from build123d import *

# Parameters (mm, degrees)
SKETCH1_W           = 13
SKETCH1_H           = 30
SKETCH1_R           = 1.8
BOSS_EXTRUDE1_DEPTH = 3
SKETCH2_W           = 13
SKETCH2_H           = 7
BOSS_EXTRUDE2_DEPTH = 31.69
SKETCH3_W           = 10
SKETCH3_H           = 14
CUT_EXTRUDE1_DEPTH  = 5.5
SKETCH4_W           = 3
SKETCH4_H           = 4
CUT_EXTRUDE2_DEPTH  = 47.940346185
FILLET1_R           = 3


with BuildPart() as part:
    # Sketch1 → Boss-Extrude1 (new body)
    with BuildSketch(Plane.XY):
        with Locations((6.5, 15)):
            Rectangle(SKETCH1_W, SKETCH1_H)
        with Locations((6.5, 25.2)):
            Circle(SKETCH1_R, mode=Mode.SUBTRACT)
        with Locations((6.5, 4.8)):
            Circle(SKETCH1_R, mode=Mode.SUBTRACT)
    extrude(amount=BOSS_EXTRUDE1_DEPTH)

    # Sketch2 → Boss-Extrude2 (add)
    with BuildSketch(Plane.XY.offset(3)):
        with Locations((6.5, 15)):
            Rectangle(SKETCH2_W, SKETCH2_H)
    extrude(amount=BOSS_EXTRUDE2_DEPTH)

    # Sketch3 → Cut-Extrude1 (cut)
    with BuildSketch(Plane(origin=(0, 18.5, 0), x_dir=(1, 0, 0), z_dir=(0, 1, 0))):
        with Locations((8, -24.69)):
            Rectangle(SKETCH3_W, SKETCH3_H)
    extrude(amount=-CUT_EXTRUDE1_DEPTH, mode=Mode.SUBTRACT)

    # Sketch4 → Cut-Extrude2 (cut, through all)
    with BuildSketch(Plane(origin=(3, 0, 0), x_dir=(0, 0, -1), z_dir=(1, 0, 0))):
        with Locations((-30.19, 15)):
            Rectangle(SKETCH4_W, SKETCH4_H)
        with Locations((-19.19, 15)):
            Rectangle(SKETCH4_W, SKETCH4_H)
    extrude(amount=-CUT_EXTRUDE2_DEPTH, mode=Mode.SUBTRACT)

    # Fillet1
    fillet1_edges = [part.edges().sort_by_distance(p)[0] for p in [
        (6.5, 11.5, 3),
        (6.5, 18.5, 3),
    ]]
    fillet(fillet1_edges, radius=FILLET1_R)


solid = part.part
CAD build for the part. Positions are in the model's coordinates, mm. A direction names the side the tool comes from. Coordinates: 2 decimals unless noted, no trailing zeros. Write each loop counter-clockwise with the first axis right and the second up, starting at its lowest first coordinate (ties: lowest second). Pieces come first, ordered by that corner, then holes. Notation, with made-up numbers: M -29,-20.75 L -17,-20.75 A33 ccw -17,15.25 Z; hole C 57,85.5 d1. An arc over 180 degrees is marked long. Answer as a JSON object with one key per item and string values. Group by question number.
1) Tool access for faces 5 (the face through (8, 27, 3)), 6 (the face through (7, 16, 31.69)), 7 (the face through (2, 15, 28.69)): list every direction of +Z, -Z, +X, -X, +Y, -Y with a clear straight run to the whole face (end or side of a thin tool).
2) Wall check: line 1 (Y direction, x = 6.5, z = 1.45); line 2 (Z direction, x = 9.5, y = 13.25); line 3 (Z direction, x = 4.75, y = 27.25). Give the ranges that are in metal, low to high. Write a range as from..to.
3) Saw through at D-D (y = 16.5). Write the cut outline in (x, z), plus the area to 3 significant figures.
4) Saw through at C-C (z = 19). Write the cut outline in (x, y), plus the area to 3 significant figures.
5) Pin check, flat tips, straight feed: pin 1 Ø3 at (x, z) = (9.5, 17.5) entering from -Y; pin 2 Ø4 at (x, y) = (8, 25) entering from +Z; pin 3 Ø4 at (x, z) = (7.5, 27.5) entering from +Y; pin 4 Ø3 at (x, y) = (6.5, 4.8) entering from +Z. Stop position of each tip, or through.
6) Mould opens along Z. For faces 1 (the face through (2, 17, 19)), 2 (the face through (6.266, 26.985, 1.479)), 3 (the face through (6, 15, 0)), 4 (the face through (6.59, 19.36, 3.9)) say: +Z half, -Z half, draft (parallel to the pull), parting line (faces both ways), or undercut.
7) Saw through at A-A (y = 25.2). Write the cut outline in (x, z).
8) Saw through at B-B (x = 6.5). Write the cut outline in (y, z), plus the area to 3 significant figures.
Values follow:
{
 "1": {"face 5": "+Z, +X, -X, +Y", "face 6": "+X", "face 7": "+X, -X"},
 "2": {"line 1": "y = 0..3, 6.6..23.4, 27..30", "line 2": "z = 0..17.69, 31.69..34.69", "line 3": "z = 0..3"},
 "3": {"outline": "M 0,0 L 13,0 L 13,17.69 L 0,17.69 Z; M 0,20.69 L 3,20.69 L 3,28.69 L 0,28.69 Z; M 0,31.69 L 13,31.69 L 13,34.69 L 0,34.69 Z", "area": "293 mm2"},
 "4": {"outline": "M 0,11.5 L 13,11.5 L 13,13 L 0,13 Z; M 0,17 L 3,17 L 3,18.5 L 0,18.5 Z", "area": "24.0 mm2"},
 "5": {"pin 1": "stops at y = 11.5", "pin 2": "stops at z = 3", "pin 3": "stops at y = 13", "pin 4": "passes through"},
 "6": {"face 1": "undercut", "face 2": "draft", "face 3": "-Z half", "face 4": "+Z half"},
 "7": {"outline": "M 0,0 L 4.7,0 L 4.7,3 L 0,3 Z; M 8.3,0 L 13,0 L 13,3 L 8.3,3 Z"},
 "8": {"outline": "M 0,0 L 3,0 L 3,3 L 0,3 Z; M 6.6,0 L 23.4,0 L 23.4,3 L 21.5,3 A3 cw 18.5,6 L 18.5,17.69 L 13,17.69 L 13,31.69 L 18.5,31.69 L 18.5,34.69 L 11.5,34.69 L 11.5,6 A3 cw 8.5,3 L 6.6,3 Z; M 27,0 L 30,0 L 30,3 L 27,3 Z", "area": "217 mm2"}
}
